CAD build for the part. Positions are in the model's coordinates, mm. Face numbers are marked on the shaded views. A direction names the side the tool comes from. Coordinates: 2 decimals unless noted, no trailing zeros. Write each loop counter-clockwise with the first axis right and the second up, starting at its lowest first coordinate (ties: lowest second). Pieces come first, ordered by that corner, then holes. Notation, with made-up numbers: (6.5, 81.5) - (47.5, 81.5) arc R18 ccw to (47.5, 115.5) - close; hole circle Ø5 at (-24.75, 81.25). An arc over 180 degrees is marked (long way). Answer in a Markdown table with one row per item. Add a question column.
Q1. Two-plate mould, pull along X, no slides. Class the marked faces 1, 2, 3 and 4: +X half, -X half, draft (parallel to the pull), parting line (faces both ways), or undercut.
Q2. 3-axis set-ups, long thin cutter, end or side, ignore diameter. For the marked faces 5 and 6: which of +Z, -Z, +X, -X, +Y, -Y reach the whole face in a straight line?
Q3. Pin check, flat tips, straight feed: pin 1 (10 mm diameter, centred on x = 23, z = -50, fed in from +Y) (3 decimals); pin 2 (6 mm diameter, centred on y = 20.64, z = -108.58, fed in from +X). Stop position of each tip, or through.
Q4. Drill centre lines: line 1 along Z through (x, y) = (42, 26.5); line 2 along X through (y, z) = (31.5, -147); line 3 along Z through (x, y) = (102.5, 23). Where is each one in solid material? Low to high. Write a range as from..to.
Q5. Band-saw the part on C-C (z = -22). List the corners of the cut face in (x, y) (3 decimals), and give its area (3 significant figures).
Q6. Band-saw the part on B-B (x = 75). List the corners of the cut face in (y, z) (3 decimals).
Q7. Band-saw the part on A-A (y = 38.5). List the corners of the cut face in (x, z) (3 decimals), and give its area (3 significant figures).
Autodesk Inventor part; units mm, degrees
ref_plane "YZ Plane" through (0, 0, 0) normal (1, 0, 0) x (0, 1, 0)
ref_plane "XZ Plane" through (0, 0, 0) normal (0, 1, 0) x (-1, 0, 0)
ref_plane "XY Plane" through (0, 0, 0) normal (0, 0, 1) x (1, 0, 0)
sketch "Sketch3" plane through (0, 0, 0) normal (0, 1, 0) x (-1, 0, 0)
  line L0 (0, 0) -> (-106.68, 0)
  line L1 (-106.68, 0) -> (-106.68, -153.67)
  line L2 (-106.68, -153.67) -> (0, -153.67)
  line L3 (0, -153.67) -> (0, 0)
  line L4 (-15.24, -138.43) -> (-91.44, -138.43) construction
  line L5 (-91.44, -138.43) -> (-91.44, -87.63) construction
  line L6 (-91.44, -87.63) -> (-15.24, -87.63) construction
  line L7 (-15.24, -87.63) -> (-15.24, -138.43) construction
  line L8 (-15.24, -66.04) -> (-91.44, -66.04) construction
  line L9 (-91.44, -66.04) -> (-91.44, -15.24) construction
  line L10 (-91.44, -15.24) -> (-15.24, -15.24) construction
  line L11 (-15.24, -15.24) -> (-15.24, -66.04) construction
  dimension "d0" = 76.2
  dimension "d1" = 50.8
  dimension "d2" = 15.24
  dimension "d3" = 15.24
  dimension "d4" = 15.24
  dimension "d5" = 15.24
  dimension "d6" = 21.59
extrude "Extrusion1" add sketch "Sketch3" along normal blind 3.175
sketch "Sketch4" plane through (0, 3.175, 0) normal (0, 1, 0) x (1, 0, 0)
  line L0 (0, 0) -> (106.68, 0)
  line L1 (106.68, 0) -> (106.68, 153.67)
  line L2 (106.68, 153.67) -> (0, 153.67)
  line L3 (0, 153.67) -> (0, 0)
  line L4 (4.826, 4.826) -> (101.854, 4.826)
  line L5 (101.854, 4.826) -> (101.854, 148.844)
  line L6 (101.854, 148.844) -> (4.826, 148.844)
  line L7 (4.826, 148.844) -> (4.826, 4.826)
  dimension "d9" = 4.826
extrude "Extrusion2" add sketch "Sketch4" along normal blind 38.1
sketch "Sketch5" plane through (0, 3.175, 0) normal (0, 1, 0) x (1, 0, 0)
  line L0 (18.9992, 137.8966) -> (87.6808, 137.8966) construction
  line L1 (87.6808, 137.8966) -> (87.6808, 15.7734) construction
  line L2 (87.6808, 15.7734) -> (18.9992, 15.7734) construction
  line L3 (18.9992, 15.7734) -> (18.9992, 137.8966) construction
  line L4 (18.9992, 15.7734) -> (87.6808, 15.7734) construction
  line L5 (87.6808, 15.7734) -> (87.6808, 64.135) construction
  line L6 (87.6808, 64.135) -> (18.9992, 64.135) construction
  line L7 (18.9992, 64.135) -> (18.9992, 15.7734) construction
  line L8 (87.6808, 137.8966) -> (18.9992, 137.8966) construction
  line L9 (18.9992, 137.8966) -> (18.9992, 89.535) construction
  line L10 (18.9992, 89.535) -> (87.6808, 89.535) construction
  line L11 (87.6808, 89.535) -> (87.6808, 137.8966) construction
  line L12 (4.826, 148.844) -> (4.826, 4.826) construction
  line L13 (4.826, 4.826) -> (101.854, 4.826) construction
  line L14 (101.854, 4.826) -> (101.854, 148.844) construction
  line L15 (101.854, 148.844) -> (4.826, 148.844) construction
  point P0 (0, 0)
  dimension "d12" = 68.6816
  dimension "d13" = 48.3616
  dimension "d14" = 48.3616
  dimension "d15" = 14.1732
  dimension "d16" = 10.9474
  dimension "d17" = 10.9474
  dimension "d18" = 14.1732
  dimension "d19" = 25.4
sketch "Sketch6" plane through (106.68, 0, 0) normal (1, 0, 0) x (0, 0, -1)
  line L0 (45.085, 20.6375) -> (108.585, 20.6375) construction
  line L1 (0, 41.275) -> (153.67, 41.275)
  line L2 (0, 0) -> (153.67, 0)
  line L3 (0, 0) -> (0, 41.275)
  line L4 (153.67, 0) -> (153.67, 41.275)
  dimension "d20" = 20.6375
  dimension "d21" = 20.6375
  dimension "d22" = 45.085
  dimension "d23" = 45.085
  dimension "d24" = 63.5
hole "Hole1" at (106.68, 20.6375, -45.085) at (106.68, 20.6375, -108.585) direction (-1, 0, 0) diameter 7.62 end up to surface
sketch "Sketch7" plane through (0, 0, -153.67) normal (-1, 0, 0) x (0, 0, 1)
  line L0 (0, 0) -> (153.67, 0)
  line L1 (0, 41.275) -> (153.67, 41.275)
  line L2 (153.67, 0) -> (153.67, 41.275)
  line L3 (0, 0) -> (0, 41.275)
  point P0 (76.835, 20.6375)
  dimension "d32" = 20.6375
  dimension "d33" = 20.6375
  dimension "d34" = 76.835
  dimension "d35" = 76.835
hole "Hole2" at (0, 20.6375, -76.835) direction (1, 0, 0) diameter 12.7 end up to surface
chamfer "Chamfer1" distance 1.27 angle 45 4 edges at (106.68, 0, -76.835) (53.34, 0, -153.67) (0, 0, -76.835) (53.34, 0, 0)
fillet "Fillet1" radius 3.175 4 edges at (106.68, 21.2725, -153.67) (106.68, 21.2725, 0) (0, 21.2725, 0) (0, 21.2725, -153.67)
sketch "Sketch8" plane through (0, 1.27, -150.495) normal (-1, 0, 0) x (0, 0, 1)
  circle A0 centre (73.66, 19.3675) radius 6.35 construction
  line L0 (68.4584, 23.0097) -> (73.66, 30.4384)
  line L1 (73.66, 30.4384) -> (78.8616, 23.0097)
  line L2 (73.66, 19.3675) -> (73.66, 30.4384) construction
  line L3 (68.4584, 23.0097) -> (78.8616, 23.0097) construction
  arc A1 (78.8616, 23.0097) -> (68.4584, 23.0097) centre (73.66, 19.3675) ccw
  point P0 (150.495, -1.27)
  dimension "d47" = 55
extrude "Extrusion3" cut sketch "Sketch8" against normal up to surface (4.826 mm away)
sketch "Sketch9" plane through (106.68, 1.27, -3.175) normal (1, 0, 0) x (0, 0, -1)
  circle A0 centre (41.91, 19.3675) radius 3.81 construction
  circle A1 centre (105.41, 19.3675) radius 3.81 construction
  line L0 (0, 0) -> (0, 40.005) construction
  line L1 (147.32, 0) -> (0, 0) construction
  line L2 (147.32, 40.005) -> (147.32, 0) construction
  line L3 (0, 40.005) -> (147.32, 40.005) construction
  line L4 (38.789, 21.5528) -> (41.91, 26.01)
  line L5 (41.91, 26.01) -> (45.031, 21.5528)
  line L6 (102.289, 21.5528) -> (105.41, 26.01)
  line L7 (105.41, 26.01) -> (108.531, 21.5528)
  circle A2 centre (41.91, 19.3675) radius 3.81
  circle A3 centre (105.41, 19.3675) radius 3.81
  line L8 (41.91, 19.3675) -> (41.91, 26.01) construction
  line L9 (105.41, 19.3675) -> (105.41, 26.01) construction
  line L10 (38.789, 21.5528) -> (45.031, 21.5528) construction
  point P0 (-3.175, -1.27)
  dimension "d50" = 55
extrude "Extrusion4" cut sketch "Sketch9" against normal up to surface (4.826 mm away) contours L4 L5 A2 | L6 L7 A3
equation "\"d3\" = d2"
equation "\"d4\" = d2"
equation "\"d5\" = d3"
equation "\"d17\" = d16"
equation "\"d18\" = d15"
equation "\"d20\" = d21"
equation "\"d23\" = d22"
properties part number "bottom"
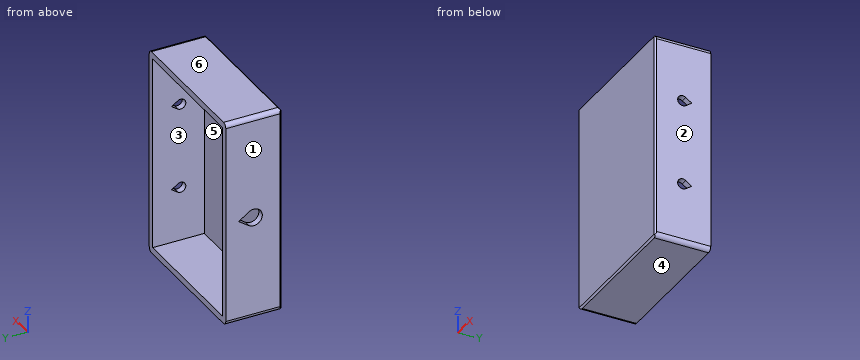
Checked values:
| question | item | result |
|---|---|---|
| 1 | face 1 | -X half |
| 1 | face 2 | +X half |
| 1 | face 3 | undercut |
| 1 | face 4 | draft |
| 2 | face 5 | +Y |
| 2 | face 6 | +Z, +X, -X, +Y, -Y |
| 3 | pin 1 | stops at y = 3.175 |
| 3 | pin 2 | stops at x = 4.83 |
| 4 | line 1 | z = -153.67..-148.84, -4.83..0 |
| 4 | line 2 | x = 0..4.83, 101.85..106.68 |
| 4 | line 3 | z = -153.67..-111.58, -105.59..-48.08, -42.09..0 |
| 5 | outline | (0, 1.27) - (1.27, 0) - (105.41, 0) - (106.68, 1.27) - (106.68, 41.275) - (101.854, 41.275) - (101.854, 3.175) - (4.826, 3.175) - (4.826, 41.275) - (0, 41.275) - close |
| 5 | area | 705 mm² |
| 6 | outline | (0, -152.4) - (1.27, -153.67) - (41.275, -153.67) - (41.275, -148.844) - (3.175, -148.844) - (3.175, -4.826) - (41.275, -4.826) - (41.275, 0) - (1.27, 0) - (0, -1.27) - close |
| 7 | outline | (0, -150.495) arc R3.175 ccw to (3.175, -153.67) - (103.505, -153.67) arc R3.175 ccw to (106.68, -150.495) - (106.68, -3.175) arc R3.175 ccw to (103.505, 0) - (3.175, 0) arc R3.175 ccw to (0, -3.175) - close; hole (4.826, -148.844) - (101.854, -148.844) - (101.854, -4.826) - (4.826, -4.826) - close |
| 7 | area | 2,410 mm² |
